Input: dimensioned drawing with shaded views. Units: mm. Origin: part minimum x, y, z. A direction names the side the tool comes from. Round coordinates to 2 decimals unless told otherwise and drop trailing zeros. Order: outer loops, then holes, each group sorted by start corner. A loop starts at its lowest first (then second) coordinate and runs counter-clockwise, first axis right, second up. Notation, with made-up numbers: M 27.5,33 L 86.5,33 A18 ccw 86.5,58 Z; hole C -10.5,-23 d4. An arc over 180 degrees is marked long. Put each result on its own line as item: value. Start each with the question number.
1) Draft query along X for the marked faces 3, 4 and 5. Return one class per face: pulls with the +X half, pulls with the -X half, needs draft (parallel to the pull), parting line crosses it, or undercut.
2) Material intervals for probe 1 along Z at (x, y) = (6, 3.5); probe 2 along X at (y, z) = (0.5, 19); probe 3 along X at (y, z) = (6, 37), sorted ascending. Write a range as [from, to].
3) Access query for the marked faces 1 and 2. Directions: +Z, -Z, +X, -X, +Y, -Y. A direction counts if a zero-diameter tool reaches every point of the face in a straight line with its end or side. Return the directions, or none.
4) Section A-A, the plane z = 17.5. Return loops of the section in (x, y).
5) Section D-D, the plane y = 4.25. Return loops of the section in (x, z), then the cut area to 3 significant figures.
6) Section C-C, the plane z = 6. Return loops of the section in (x, y).
7) Section B-B, the plane x = 74. Return loops of the section in (y, z).
8) First-contact query: P1, Ø5.5, axis at x = 6, z = 6, coming from the -Y side. Flat tip, straight axial feed; report the tip coordinate or a pass-through.
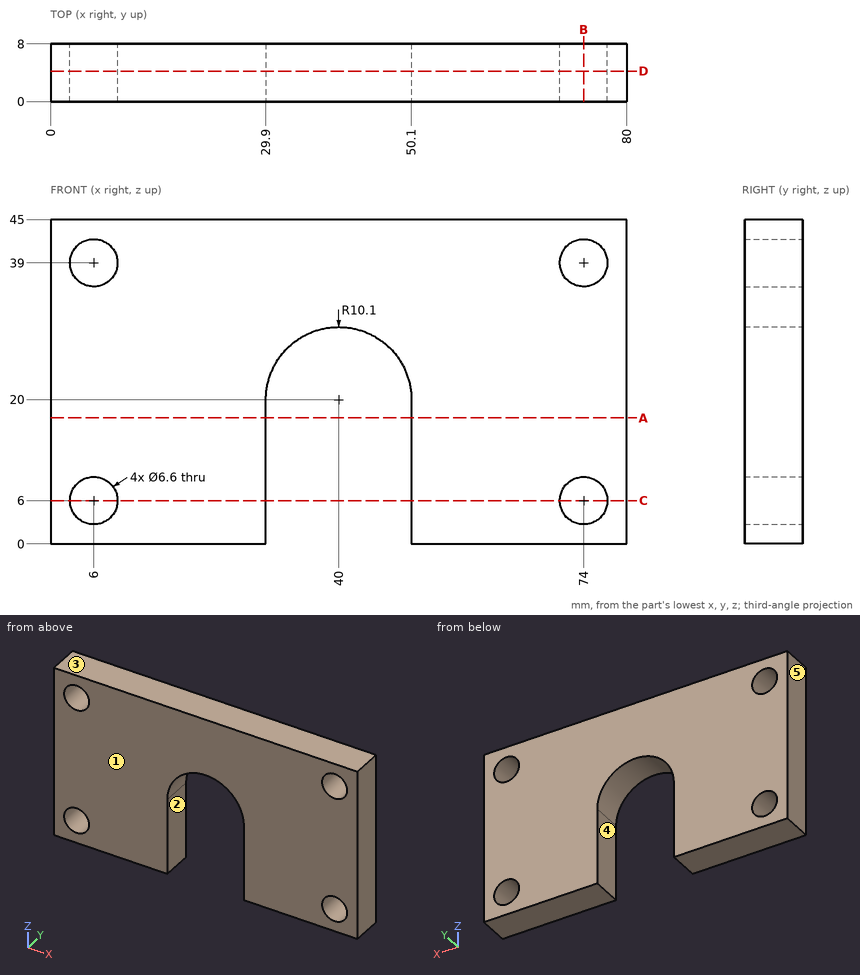
Result sheet:
1. face 3: needs draft
1. face 4: undercut
1. face 5: pulls with the -X half
2. probe 1: z = [0, 2.7], [9.3, 35.7], [42.3, 45]
2. probe 2: x = [0, 29.9], [50.1, 80]
2. probe 3: x = [0, 3.38], [8.62, 71.38], [76.62, 80]
3. face 1: +Z, -Z, +X, -X, -Y
3. face 2: -Z, +Y, -Y
4. outline: M 0,0 L 29.9,0 L 29.9,8 L 0,8 Z; M 50.1,0 L 80,0 L 80,8 L 50.1,8 Z
5. outline: M 0,0 L 29.9,0 L 29.9,20 A10.1 cw 50.1,20 L 50.1,0 L 80,0 L 80,45 L 0,45 Z; hole C 6,6 d6.6; hole C 6,39 d6.6; hole C 74,6 d6.6; hole C 74,39 d6.6
5. area: 2,900 mm2
6. outline: M 0,0 L 2.7,0 L 2.7,8 L 0,8 Z; M 9.3,0 L 29.9,0 L 29.9,8 L 9.3,8 Z; M 50.1,0 L 70.7,0 L 70.7,8 L 50.1,8 Z; M 77.3,0 L 80,0 L 80,8 L 77.3,8 Z
7. outline: M 0,0 L 8,0 L 8,2.7 L 0,2.7 Z; M 0,9.3 L 8,9.3 L 8,35.7 L 0,35.7 Z; M 0,42.3 L 8,42.3 L 8,45 L 0,45 Z
8. P1: passes through
